Geometry check sheet. Reference: the model listing, model coordinates, mm. Face numbers are marked on the shaded views. Coordinates: 2 decimals unless noted, no trailing zeros. Write each loop counter-clockwise with the first axis right and the second up, starting at its lowest first coordinate (ties: lowest second). Pieces come first, ordered by that corner, then holes. Notation, with made-up numbers: (89, -5) -> (97, -5) arc R13 cw to (97, 6) -> close; hole circle Ø7 at (30, 62.25). An arc over 180 degrees is marked (long way). Use a Markdown table: item, result.
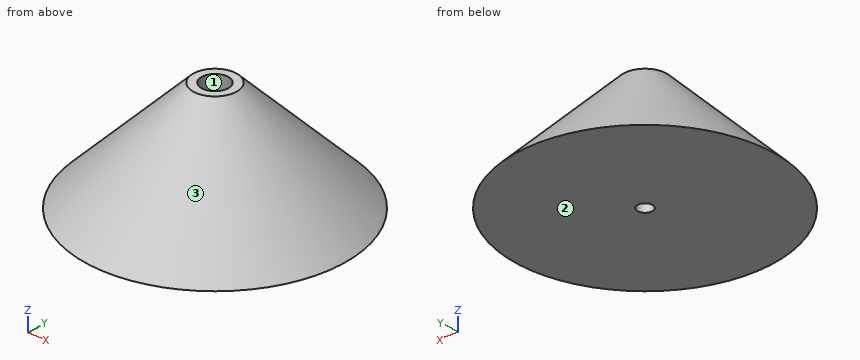
```python
from build123d import *

# Parameters (mm, degrees)
F0_R           = 152.4
F1_DEPTH       = 127
F3_D           = 17.5
F3_CBORE_D     = 31.5
F3_CBORE_DEPTH = 20
F4_SIZE        = 126.99999


# Not quite as in the source:
# - a fillet or chamfer is up to 0.001 mm smaller than in the source, because OpenCascade refuses the exact size


with BuildPart() as f1:
    # F0 (on Top) → F1 (new body)
    with BuildSketch(Plane.XY):
        Circle(F0_R)
    extrude(amount=F1_DEPTH)

    # F3 (through all)
    with Locations(Plane.XY.offset(127)):
        with Locations((0, 0)):
            CounterBoreHole(F3_D / 2, F3_CBORE_D / 2, F3_CBORE_DEPTH)

    # F4 (size 127 in the source; OpenCascade refuses exactly that, so slightly less here)
    f4_edges = [f1.edges().sort_by_distance(p)[0] for p in [
        (-152.4, 0, 127),
    ]]
    chamfer(f4_edges, length=F4_SIZE)


solid = f1.part
```
Item 1: Depth check by flat-ended pin: P1, Ø6, axis at x = -89, y = 8, coming from the +Z side; P2, Ø1.5, axis at y = 67.5, z = 37, coming from the -X side; P3, Ø12, axis at x = -46.5, y = 86, coming from the -Z side; P4, Ø1.5, axis at x = 42.5, y = 87.5, coming from the +Z side. Enter the tip coordinate at first touch or a pass-through.
Answer block:
| item | result |
|---|---|
| P1 | stops at z = 66.04 |
| P2 | stops at x = -94.67 |
| P3 | stops at z = 0 |
| P4 | stops at z = 55.87 |
Item 2: Mould release check, pull along X, two halves, no side actions. Record for the marked faces 1, 2 and 3: +X half, -X half, draft (parallel to the pull), parting line (faces both ways), or undercut.
Answer block:
| item | result |
|---|---|
| face 1 | undercut |
| face 2 | draft |
| face 3 | parting line |
Item 3: Section check C-C on z = 78. Record the boundary of the cut face in (x, y), then the cut area to 3 significant figures.
Answer block:
| item | result |
|---|---|
| outline | circle Ø148.8 at (0, 0); hole circle Ø17.5 at (0, 0) |
| area | 17,100 mm^2 |
Item 4: Thickness scan on L1, parallel to Y at x = 0, z = 73; L2, parallel to Y at x = 0, z = 51; L3, parallel to Z at x = 91, y = 73.5. Record the ranges inside material, lowest first. Write a range as [from, to].
Answer block:
| item | result |
|---|---|
| L1 | y = [-79.4, -8.75], [8.75, 79.4] |
| L2 | y = [-101.4, -8.75], [8.75, 101.4] |
| L3 | z = [0, 35.42] |
Item 5: Section check D-D on z = 50. Record the boundary of the cut face in (x, y).
Answer block:
| item | result |
|---|---|
| outline | circle Ø204.8 at (0, 0); hole circle Ø17.5 at (0, 0) |
